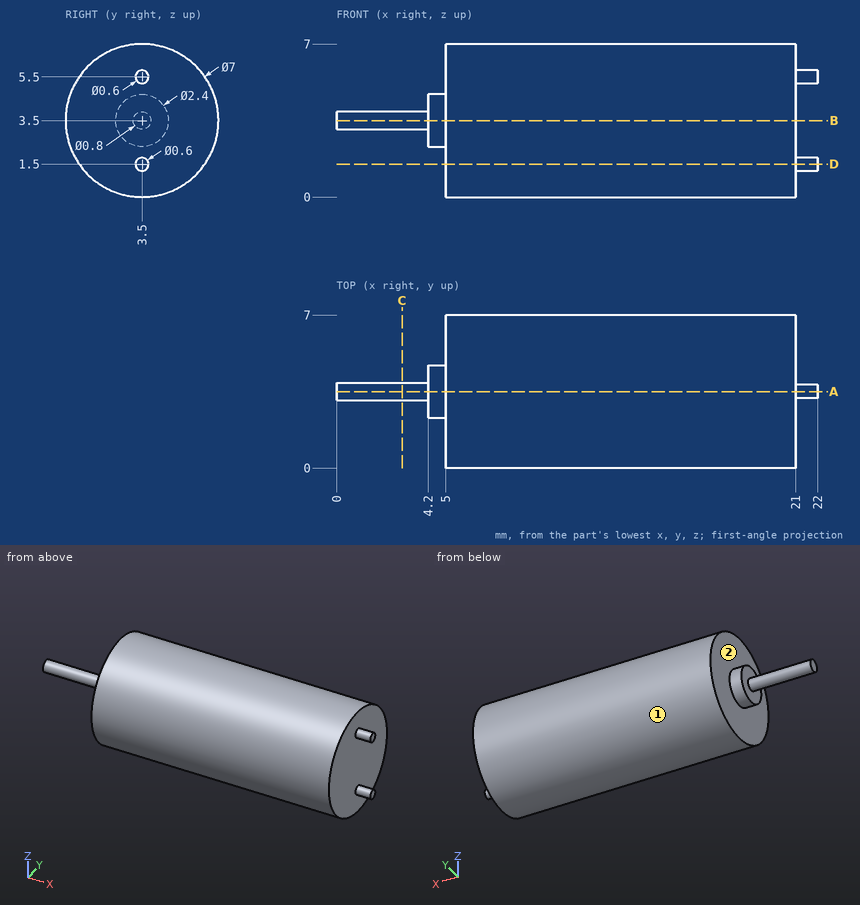
Design review of the part shown in the three views and the two pictorial views. Dimensions are in mm from the part's minimum x, y and z. A direction names the side the tool comes from. Give positions to 0.01 mm unless a question says otherwise; leave off trailing zeros. Write each loop counter-clockwise with the first axis right and the second up, starting at its lowest first coordinate (ties: lowest second). Pieces come first, ordered by that corner, then holes.
Item 1: Take a section at A-A (y = 3.5). Give the boundary of the cut face in (x, z).
Item 2: Insertion check: P1, Ø2, axis at y = 4.5, z = 4, coming from the +X side; P2, Ø1.5, axis at x = 5, z = 1, coming from the -Y side; P3, Ø1.5, axis at x = 3, y = 0.5, coming from the +Z side. Each pin has a flat end and moves straight along its axis. Give the tip position at first contact, or say it passes through.
Item 3: Machinability: for the marked faces 1 and 2, which of the approach directions +Z, -Z, +X, -X, +Y, -Y give a long, thin tool a straight path to every point of the face, cutting with its end or side? Answer none if there is none.
Item 4: Take a section at D-D (z = 1.5). Give the boundary of the cut face in (x, y).
Item 5: Take a section at C-C (x = 3). Give the boundary of the cut face in (y, z).
Item 6: Wall thickness on probe 1 along X at (y, z) = (4, 2.5); probe 2 along Y at (x, z) = (21.25, 1.5); probe 3 along X at (y, z) = (4.75, 1.5): over which ranges is each line inside the solid? List them lowest first.
Item 7: Take a section at B-B (z = 3.5). Give the boundary of the cut face in (x, y).
Established:
1. outline: (0, 3.1) - (4.2, 3.1) - (4.2, 2.3) - (5, 2.3) - (5, 0) - (21, 0) - (21, 1.2) - (22, 1.2) - (22, 1.8) - (21, 1.8) - (21, 5.2) - (22, 5.2) - (22, 5.8) - (21, 5.8) - (21, 7) - (5, 7) - (5, 4.7) - (4.2, 4.7) - (4.2, 3.9) - (0, 3.9) - close
2. P1: stops at x = 21
2. P2: stops at y = 0.47
2. P3: passes through
3. face 1: +X, -X
3. face 2: -X
4. outline: (5, 0.63) - (21, 0.63) - (21, 3.2) - (22, 3.2) - (22, 3.8) - (21, 3.8) - (21, 6.37) - (5, 6.37) - close
5. outline: circle Ø0.8 at (3.5, 3.5)
6. probe 1: x = 4.2 to 21
6. probe 2: y = 3.2 to 3.8
6. probe 3: x = 5 to 21
7. outline: (0, 3.1) - (4.2, 3.1) - (4.2, 2.3) - (5, 2.3) - (5, 0) - (21, 0) - (21, 7) - (5, 7) - (5, 4.7) - (4.2, 4.7) - (4.2, 3.9) - (0, 3.9) - close
